CAD build for the part. Positions are in the model's coordinates, mm. A direction names the side the tool comes from. Round coordinates to 2 decimals unless told otherwise and drop trailing zeros. Loops run counter-clockwise (first coordinate to the right, second up) from the corner with the lowest first, then second, coordinate; pieces in that order, holes last. Notation, with made-up numbers: (-8.5, -0.75) - (16.5, -0.75) arc R26 ccw to (16.5, 37.25) - close; hole circle Ø2 at (63.5, -13.75). An arc over 180 degrees is marked (long way). One line per question, with ' | ' between items.
Autodesk Inventor part; units mm, degrees
ref_plane "YZ Plane" through (0, 0, 0) normal (1, 0, 0) x (0, 1, 0)
ref_plane "XZ Plane" through (0, 0, 0) normal (0, 1, 0) x (-1, 0, 0)
ref_plane "XY Plane" through (0, 0, 0) normal (0, 0, 1) x (1, 0, 0)
sketch "Sketch1" plane through (0, 0, 0) normal (0, 0, 1) x (1, 0, 0)
  line L0 (25, -19) -> (-25, -19)
  line L1 (-25, 31) -> (25, 31)
  line L2 (25, 31) -> (25, -69)
  line L3 (25, -69) -> (-25, -69)
  line L4 (-25, -69) -> (-25, 31)
  line L5 (-25, 31) -> (25, -69) construction
  line L6 (25, 31) -> (-25, -69) construction
  line L7 (25, -69) -> (-25, -69)
  line L8 (-25, -69) -> (-25, -119)
  line L9 (-25, -119) -> (25, -119)
  line L10 (25, -119) -> (25, -69)
  point P0 (0, 0)
  point P1 (0, -19)
  dimension "d0" = 50
  dimension "d1" = 100
  dimension "d2" = 50
  dimension "d3" = 50
extrude "Extrusion1" add sketch "Sketch1" along normal blind 5
fillet "Fillet1" radius 10 2 edges at (25, -119, 2.5) (-25, -119, 2.5)
ref_plane "Work Plane1" through (-15, -19, 0) normal (0, -1, 0) x (1, 0, 0)
sketch "Sketch2" plane through (-15, -19, 0) normal (0, -1, 0) x (1, 0, 0)
  line L0 (40, -0.5) -> (-10, -0.5)
  line L1 (-10, -0.5) -> (-10, -3.5)
  line L2 (40, -3.5) -> (-10, -3.5)
  line L3 (40, -0.5) -> (40, -3.5)
  line L4 (-10, -3.5) -> (40, -3.5)
  line L5 (-10, -3.5) -> (-10, -53.5)
  line L6 (-10, -53.5) -> (40, -53.5)
  line L7 (40, -53.5) -> (40, -3.5)
  line L8 (40, -3.5) -> (-10, -3.5)
  ellipse E0 centre (15, -28.5) end of major axis (18.5, -28.5) minor radius 3.5
  line L9 (-10, 0) -> (0, 0)
  line L10 (40, 0) -> (-10, 0)
  line L11 (30, 0) -> (40, 0)
  line L12 (0, 0) -> (30, 0)
  line L13 (25, -0.5) -> (5, -0.5)
  line L14 (5, -0.5) -> (5, -20.5)
  line L15 (25, -20.5) -> (5, -20.5)
  line L16 (25, -0.5) -> (25, -20.5)
  line L17 (40, 0) -> (28, 0)
  line L18 (28, 0) -> (28, -20)
  line L19 (28, -20) -> (40, -20)
  line L20 (40, -20) -> (40, 0)
  line L21 (-10, 0) -> (2, 0)
  line L22 (2, 0) -> (2, -20)
  line L23 (2, -20) -> (-10, -20)
  line L24 (-10, -20) -> (-10, 0)
  point P0 (15, 0)
  dimension "d8" = 12
  dimension "d9" = 20
  dimension "d10" = 12
  dimension "d11" = 20
extrude "Extrusion2" add sketch "Sketch2" along normal blind 20 contours L18 L10 L20 L0 | L0 L3 L2 L18 | L22 L2 L1 L0 | L0 L24 L9 L10 L22 | L2 L7 L19 L18 | L22 L23 L5 L2
chamfer "Chamfer1" distance 15 angle 45 2 edges at (-19, -39, -20) (19, -39, -20)
fillet "Fillet2" radius 10 2 edges at (-19, -24, -20) (-19, -39, -5)
fillet "Fillet3" radius 10 2 edges at (19, -39, -5) (19, -24, -20)
sketch "Sketch3" plane through (0, 0, 5) normal (0, 0, 1) x (1, 0, 0)
  line L0 (25, -109) -> (25, 31)
  line L1 (-25, 31) -> (-25, -109)
  line L2 (25, 31) -> (-25, 31)
  line L3 (-25, 31) -> (-25, -19)
  line L4 (-25, -19) -> (25, -19)
  line L5 (25, -19) -> (25, 31)
  line L6 (-15, 51) -> (15, 51)
  line L7 (15, 51) -> (15, 21)
  line L8 (15, 21) -> (-15, 21)
  line L9 (-15, 21) -> (-15, 51)
  line L10 (-15, 51) -> (15, 21) construction
  line L11 (15, 51) -> (-15, 21) construction
  circle A0 centre (15, 21) radius 1.5
  circle A1 centre (15, 51) radius 1.5
  circle A2 centre (-15, 51) radius 1.5
  circle A3 centre (-15, 21) radius 1.5
  point P0 (0, 0)
  point P1 (0, 36)
  dimension "d19" = 50
  dimension "d20" = 30
  dimension "d21" = 30
  dimension "d22" = 3
  dimension "d23" = 3
  dimension "d24" = 3
  dimension "d25" = 3
extrude "Extrusion3" cut sketch "Sketch3" against normal blind 20 contours A1 L6 L7 | L7 L6 A1 | A0 L8 L7 | L7 L8 A0 | A3 L8 L9 | L9 L8 A3 | A2 L6 L9 | L9 L6 A2
sketch "Sketch4" plane through (-15, -19, 0) normal (0, 1, 0) x (1, 0, 0)
  line L0 (-10, 0) -> (-10, 20)
  line L1 (-10, 20) -> (2, 20)
  line L2 (2, 20) -> (2, 8)
  line L3 (2, 8) -> (-10, 8)
  line L4 (-10, 8) -> (-10, 20)
  circle A0 centre (-4, 14) radius 1.5
  circle A1 centre (34, 14) radius 1.5
  point P0 (15, 0)
  dimension "d28" = 12
  dimension "d29" = 12
  dimension "d30" = 3
  dimension "d33" = 38
extrude "Extrusion4" cut sketch "Sketch4" against normal through all contours A0 | A1
sketch "Sketch5" plane through (-15, -39, 0) normal (0, -1, 0) x (1, 0, 0)
  circle A0 centre (34, -14) radius 1.5
  circle A1 centre (-4, -14) radius 1.5
  circle A2 centre (34, -14) radius 2.5
  circle A3 centre (-4, -14) radius 1.5
  circle A4 centre (-4, -14) radius 2.5
  point P0 (15, 0)
  dimension "d40" = 5
  dimension "d41" = 5
extrude "Extrusion5" cut sketch "Sketch5" against normal blind 15
sketch "Sketch6" plane through (0, 0, 0) normal (0, 0, -1) x (-1, 0, 0)
  circle A0 centre (0, -55) radius 5
  circle A1 centre (0, -38.75) radius 2.6
  circle A2 centre (0, -71.25) radius 2.6
  point P0 (0, 0)
  dimension "d44" = 10
  dimension "d45" = 16.25
  dimension "d46" = 16.25
  dimension "d47" = 5.2
  dimension "d48" = 5.2
  dimension "d51" = 55
extrude "Extrusion6" cut sketch "Sketch6" against normal blind 15
sketch "Sketch7" plane through (0, 0, 0) normal (0, 0, -1) x (-1, 0, 0)
  line L0 (25, 31) -> (25, -109)
  line L1 (25, -84) -> (-25, -84)
  line L2 (-25, -109) -> (-25, 31)
  line L3 (25, -84) -> (75, -84) construction
  line L4 (15, -119) -> (-15, -119)
  circle A0 centre (0, -71.25) radius 2.6
  circle A1 centre (0, -38.75) radius 2.6
  circle A2 centre (0, -55) radius 5
  circle A3 centre (15, 21) radius 1.5
  circle A4 centre (-15, 21) radius 1.5
  line L5 (-13, -39) -> (-25, -39)
  line L6 (-25, -109) -> (-25, -39)
  arc A5 (-25, -109) -> (-15, -119) centre (-15, -109) ccw
  line L7 (15, -119) -> (-15, -119)
  arc A6 (15, -119) -> (25, -109) centre (15, -109) ccw
  line L8 (25, -39) -> (25, -109)
  line L9 (25, -39) -> (13, -39)
  line L10 (13, -39) -> (13, -19)
  line L11 (13, -19) -> (25, -19)
  line L12 (25, 31) -> (25, -19)
  line L13 (-25, 31) -> (25, 31)
  line L14 (-25, -19) -> (-25, 31)
  line L15 (-25, -19) -> (-13, -19)
  line L16 (-13, -19) -> (-13, -39)
  point P0 (0, 0)
  point P1 (-15, -119)
  point P2 (15, -119)
  dimension "d52" = 50
  dimension "d53" = 180
  dimension "d54" = 35
extrude "Extrusion7" cut sketch "Sketch7" against normal blind 15 contours L0 L9 L10 L11 | L15 L16 L5 L2 | L0 A6 L4 A5 L2 L1
fillet "Fillet4" radius 10 2 edges at (25, -84, 2.5) (-25, -84, 2.5)
sketch "Sketch8" plane through (13, -19, 0) normal (0, -1, 0) x (1, 0, 0)
  line L0 (0, 5) -> (12, 5)
  line L1 (0, 0) -> (0, 5)
  line L2 (12, 0) -> (0, 0)
  line L3 (12, 5) -> (12, 0)
  line L4 (-38, 5) -> (-26, 5)
  line L5 (-38, 0) -> (-38, 5)
  line L6 (-26, 0) -> (-38, 0)
  line L7 (-26, 0) -> (-26, 5)
  point P0 (-13, 0)
extrude "Extrusion8" add sketch "Sketch8" along normal up to surface (20 mm away)
sketch "Sketch9" plane through (0, 0, 5) normal (0, 0, 1) x (1, 0, 0)
  circle A0 centre (15, 21) radius 1.5
  line L0 (15, 21) -> (-15, 21)
  line L1 (-15, 21) -> (-15, -9)
  line L2 (-15, -9) -> (15, -9)
  line L3 (15, -9) -> (15, 21)
  circle A1 centre (15, -9) radius 1.5
  circle A2 centre (-15, -9) radius 1.5
  point P0 (0, 0)
  dimension "d60" = 30
  dimension "d61" = 3
  dimension "d62" = 3
extrude "Extrusion9" cut sketch "Sketch9" against normal through all contours A1 L2 L3 | L3 L2 A1 | A2 L2 L1 | L1 L2 A2
properties part number "3d mount for linear bearing"
(1) Drop flat-ended pins along their axis: P1, Ø4, axis at x = 15, y = -9, coming from the -Z side; P2, Ø4, axis at x = -19, z = -14, coming from the -Y side; P3, Ø5.5, axis at x = -18, z = -13.5, coming from the -Y side; P4, Ø1.8, axis at x = -15, y = -9, coming from the +Z side. Give the stop position or say it passes through.
Results found:
P1: stops at z = 0 | P2: stops at y = -24 | P3: stops at y = -33.25 | P4: passes through
(2) Tool access for faces 1 (the face through (0, -26, 0)), 2 (the face through (18.67, -27.37, -11.52)), 3 (the face through (-13, -27, -8)): list every direction of +Z, -Z, +X, -X, +Y, -Y with a clear straight run to the whole face (end or side of a thin tool).
Results found:
face 1: -Z | face 2: -Y | face 3: -Z, +Y, -Y
(3) Probe L1, parallel to X at y = -9, z = 1.75; L2, parallel to X at y = -27.5, z = -14; L3, parallel to Y at x = 15, z = 2.6. List the from-to ranges inside material, lowest first.
Results found:
L1: x = -25 to -16.5, -13.5 to 13.5, 16.5 to 25 | L2: x = -25 to -21.5, -16.5 to -13, 13 to 16.5, 21.5 to 25 | L3: y = -84 to -10.5, -7.5 to 19.5, 22.5 to 31
(4) Cut at C-C, the plane x = -19. Write the cut outline in (y, z).
Results found:
outline: (-83.17, 0) - (-39, 0) - (-39, -0.86) arc R10 ccw to (-36.07, -7.93) - (-32.5, -11.5) - (-24, -11.5) - (-24, -12.5) - (-19, -12.5) - (-19, 0) - (31, 0) - (31, 5) - (-83.17, 5) - close; (-27.5, -16.5) - (-26.93, -17.07) arc R10 ccw to (-19.86, -20) - (-19, -20) - (-19, -15.5) - (-24, -15.5) - (-24, -16.5) - close
(5) Cut at D-D, the plane y = -9. Write the cut outline in (x, z).
Results found:
outline: (-25, 0) - (-16.5, 0) - (-16.5, 5) - (-25, 5) - close; (-13.5, 0) - (13.5, 0) - (13.5, 5) - (-13.5, 5) - close; (16.5, 0) - (25, 0) - (25, 5) - (16.5, 5) - close
(6) Cut at B-B, the plane z = -14. Write the cut outline in (x, y), then the cut area to 3 significant figures.
Results found:
outline: (-25, -30) - (-21.5, -30) - (-21.5, -24) - (-20.5, -24) - (-20.5, -19) - (-25, -19) - close; (-17.5, -24) - (-16.5, -24) - (-16.5, -30) - (-13, -30) - (-13, -19) - (-17.5, -19) - close; (13, -30) - (16.5, -30) - (16.5, -24) - (17.5, -24) - (17.5, -19) - (13, -19) - close; (20.5, -24) - (21.5, -24) - (21.5, -30) - (25, -30) - (25, -19) - (20.5, -19) - close | area: 174 mm²
(7) Two-plate mould, pull along X, no slides. Class faces 4 (the face through (0, 31, 2)), 5 (the face through (25, -21, -1)), 6 (the face through (13.8, -9.9, 2.5)): released by +X, released by -X, zero draft, split by the parting line, or undercut.
Results found:
face 4: zero draft | face 5: released by +X | face 6: undercut
(8) Cut at A-A, the plane y = -55. Write the cut outline in (x, z).
Results found:
outline: (-25, 0) - (-5, 0) - (-5, 5) - (-25, 5) - close; (5, 0) - (25, 0) - (25, 5) - (5, 5) - close
